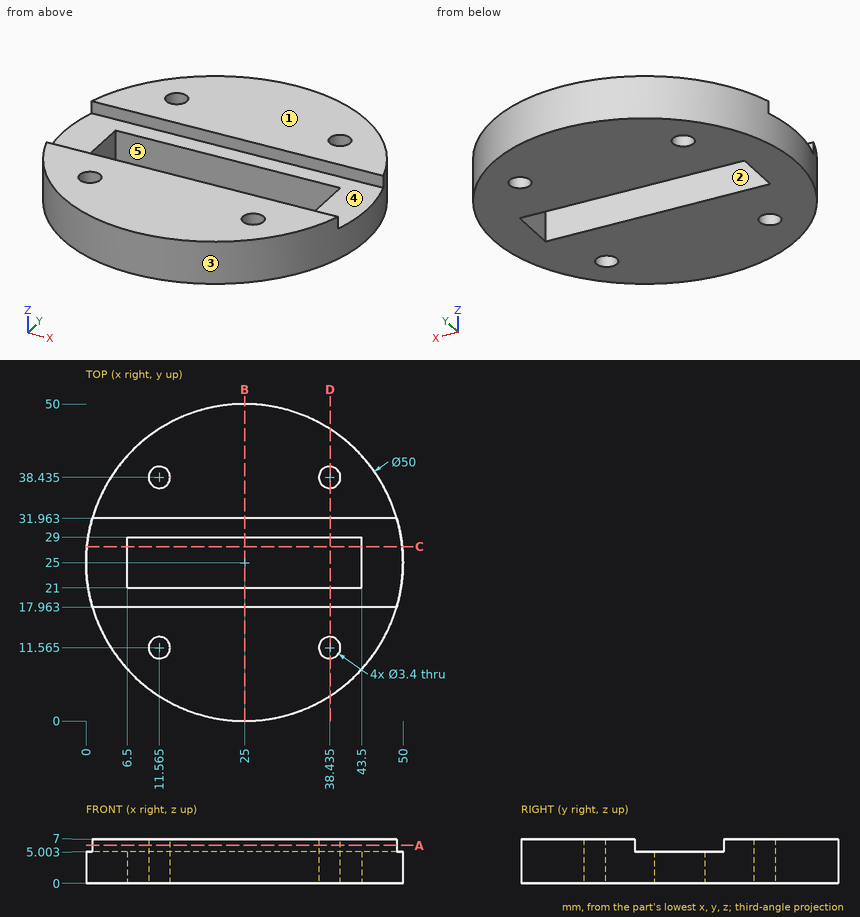
Can you work these out from the drawing? Everything is in mm from the part's minimum corner. A direction names the side the tool comes from. Coordinates: 2 decimals unless noted, no trailing zeros. Order: outer loops, then holes, each group sorted by start corner. A loop starts at its lowest first (then second) coordinate and runs counter-clockwise, first axis right, second up. Notation, with made-up numbers: (46, -9) -> (99, -9) arc R9 cw to (99, -4) -> close; hole circle Ø11 at (2.5, 40). An arc over 180 degrees is marked (long way). Return JSON: item names as keys, results as strings.
1) Thinking about a two-plate mould opening in X: for the marked faces 3, 4 and 5, which applies, +X half, -X half, draft (parallel to the pull), parting line (faces both ways), or undercut?
Conclusion:
{"face 3": "parting line", "face 4": "draft", "face 5": "undercut"}
2) If we section it at C-C on y = 27.5: List the corners of the cut face in (x, z) for me (1 decimal).
Conclusion:
{"outline": "(0.1, 0) -> (6.5, 0) -> (6.5, 5) -> (0.1, 5) -> close; (43.5, 0) -> (49.9, 0) -> (49.9, 5) -> (43.5, 5) -> close"}
3) If I drill on probe 1 along Y at (x, z) = (25.5, 1) (1 decimal); probe 2 along Y at (x, z) = (10.5, 4.25) (1 decimal); probe 3 along Y at (x, z) = (26, 6), over which ranges is the centre line in solid material (lowest first)?
Conclusion:
{"probe 1": "y = 0 to 21, 29 to 50", "probe 2": "y = 4.6 to 10.2, 12.9 to 21, 29 to 37.1, 39.8 to 45.4", "probe 3": "y = 0.02 to 17.96, 31.96 to 49.98"}
4) I'm going to push flat-ended pins straight in: P1, Ø1, axis at x = 14.5, z = 6.5, coming from the -Y side; P2, Ø4, axis at x = 27.5, z = 5, coming from the -Y side (1 decimal); P3, Ø2.5, axis at x = 22.5, z = 3, coming from the +Y side. Where does each tip first touch, or does it pass through?
Conclusion:
{"P1": "stops at y = 2.09", "P2": "stops at y = 0", "P3": "stops at y = 49.97"}
5) If we section it at A-A on z = 6: List the corners of the cut face in (x, y) for me (1 decimal).
Conclusion:
{"outline": "(1, 18) arc R25 ccw to (49, 18) -> close; (1, 32) -> (49, 32) arc R25 ccw to start; hole circle Ø3.4 at (11.6, 11.6); hole circle Ø3.4 at (11.6, 38.4); hole circle Ø3.4 at (38.4, 11.6); hole circle Ø3.4 at (38.4, 38.4)"}
6) If we section it at D-D on x = 38.5: List the corners of the cut face in (y, z) for me.
Conclusion:
{"outline": "(3.96, 0) -> (9.87, 0) -> (9.87, 7) -> (3.96, 7) -> close; (13.26, 0) -> (21, 0) -> (21, 5) -> (17.96, 5) -> (17.96, 7) -> (13.26, 7) -> close; (29, 0) -> (36.74, 0) -> (36.74, 7) -> (31.96, 7) -> (31.96, 5) -> (29, 5) -> close; (40.13, 0) -> (46.04, 0) -> (46.04, 7) -> (40.13, 7) -> close"}
7) On a 3-axis mill with a long thin cutter (end or side, diameter ignored), from which of +Z, -Z, +X, -X, +Y, -Y can I reach the whole of each face in a straight line? I mean the marked faces 1 and 2. Say none if no direction works.
Conclusion:
{"face 1": "+Z, +X, -X, +Y, -Y", "face 2": "+Z, -Z"}
8) If we section it at B-B on x = 25: List the corners of the cut face in (y, z) for me.
Conclusion:
{"outline": "(0, 0) -> (21, 0) -> (21, 5) -> (17.96, 5) -> (17.96, 7) -> (0, 7) -> close; (29, 0) -> (50, 0) -> (50, 7) -> (31.96, 7) -> (31.96, 5) -> (29, 5) -> close"}
